from build123d import *

# Parameters (mm, degrees)
CROQUIS1_W              = 237
CROQUIS1_H              = 40
CROQUIS1_W_2            = 32.55
CROQUIS1_H_2            = 30
SALIENTE_EXTRUIR1_DEPTH = 5
SALIENTE_EXTRUIR2_DEPTH = 3
REDONDEO1_R             = 10
REDONDEO2_R             = 5


with BuildPart() as part:
    # Croquis1 → Saliente-Extruir1 (new body)
    with BuildSketch(Plane.XY):
        Polygon((254.2, -311), (254.2, -341), (284.2, -341), (284.2, -381), (314.2, -381), (314.2, -311), align=None)
        Polygon((191.65, -341), (221.65, -341), (221.65, -311), (161.65, -311), (161.65, -381), (191.65, -381), align=None)
        with Locations((243.5, -401)):
            Rectangle(CROQUIS1_W, CROQUIS1_H)
        with Locations((237.925, -326)):
            Rectangle(CROQUIS1_W_2, CROQUIS1_H_2)
    extrude(amount=SALIENTE_EXTRUIR1_DEPTH)

    # Croquis1<3> → Saliente-Extruir2 (add)
    with BuildSketch(Plane.XY):
        Polygon((254.2, -311), (254.2, -341), (284.2, -341), (284.2, -381), (314.2, -381), (314.2, -311), align=None)
        Polygon((191.65, -341), (221.65, -341), (221.65, -311), (161.65, -311), (161.65, -381), (191.65, -381), align=None)
    extrude(amount=-SALIENTE_EXTRUIR2_DEPTH)

    # Redondeo1
    redondeo1_edges = [part.edges().sort_by_distance(p)[0] for p in [
        (314.2, -381, 2.5),
        (362, -381, 2.5),
        (362, -421, 2.5),
        (125, -421, 2.5),
        (125, -381, 2.5),
        (161.65, -381, 2.5),
        (161.65, -311, 1),
        (314.2, -311, 1),
        (191.65, -381, 2.5),
        (284.2, -381, 2.5),
        (284.2, -341, 1),
        (191.65, -341, 1),
    ]]
    fillet(redondeo1_edges, radius=REDONDEO1_R)

    # Redondeo2
    redondeo2_edges = [part.edges().sort_by_distance(p)[0] for p in [
        (314.2, -381, -1.5),
        (284.2, -381, -1.5),
        (254.2, -341, -1.5),
        (254.2, -311, -1.5),
        (221.65, -341, -1.5),
        (221.65, -311, -1.5),
        (161.65, -381, -1.5),
        (191.65, -381, -1.5),
    ]]
    fillet(redondeo2_edges, radius=REDONDEO2_R)


solid = part.part
Work out the finished part from the listing and answer in its coordinate system (mm). A direction names the side the tool comes from. Round coordinates to 2 decimals unless told otherwise and drop trailing zeros. Order: outer loops, then holes, each group sorted by start corner. A loop starts at its lowest first (then second) coordinate and runs counter-clockwise, first axis right, second up. Notation, with made-up numbers: M 0.5,87.5 L 29.5,87.5 A10 ccw 29.5,101.5 Z; hole C -10,-12 d9. An arc over 180 degrees is marked long. Put each result on its own line as item: value. Start each with the question number.
Q1. Section D-D, the plane y = -408 is taken. Write down the section's boundary in (x, z), and give its area (4 significant figures).
Q2. Straight lines are drawn through the part: L1, parallel to X at y = -359, z = -2.25; L2, parallel to Y at x = 211.5, z = 1; L3, parallel to X at y = -333.5, z = -1. For each, find the intervals that lie inside material, in ascending order. Write a range as [from, to].
Q3. A tool of negligible diameter and unlimited length cuts with its end or side. For faces 1 (the cylindrical face through (190.22, -379.5, -1.52)), 2 (the cylindrical face through (358.99, -383.85, 2.54)), 3 (the cylindrical face through (281.35, -344.01, 1.06)), 4 (the flat face through (125, -401, 2)), 5 (the flat face through (143, -381, 2)), from which of +Z, -Z, +X, -X, +Y, -Y can it reach the whole face along a straight path? Write none if from no direction.
Q4. Flat-ended cylindrical pins translate along their axes: pin 1 (0.9 mm diameter, centred on y = -330.5, z = -1, fed in from -X); pin 2 (0.9 mm diameter, centred on x = 176.5, z = -1, fed in from -Y); pin 3 (1.5 mm diameter, centred on x = 343, z = 1.5, fed in from +Y). Find the tip coordinate at first contact, or state that the pin passes through.
Q5. Section B-B, the plane y = -360.5 is taken. Write down the section's boundary in (x, z).
Q6. Section C-C, the plane x = 342 is taken. Write down the section's boundary in (y, z).
Q7. For a pull along X with two mould halves and no side action, classify faces 6 (the flat face through (290, -338, -3)), 7 (the cylindrical face through (255.63, -312.5, -1.52)), 8 (the cylindrical face through (358.99, -418.15, 2.54)) as pulls with the +X half, pulls with the -X half, needs draft (parallel to the pull), parting line crosses it, or undercut.
Q8. Section A-A, the plane z = -1.5 is taken. Write down the section's boundary in (x, y), and give its area (3 significant figures).
Findings below:
1. outline: M 125,0 L 362,0 L 362,5 L 125,5 Z
1. area: 1,185 mm^2
2. L1: x = [161.65, 191.65], [284.2, 314.2]
2. L2: y = [-421, -381], [-341, -311]
2. L3: x = [161.65, 221.65], [254.2, 314.2]
3. face 1: -Z, -Y
3. face 2: +Z, -Z, +X, +Y
3. face 3: +Z, -Z
3. face 4: +Z, -Z, -X, +Y, -Y
3. face 5: +Z, -Z, -X, +Y
4. pin 1: stops at x = 161.65
4. pin 2: stops at y = -381
4. pin 3: stops at y = -381
5. outline: M 161.65,-3 L 191.65,-3 L 191.65,5 L 161.65,5 Z; M 284.2,-3 L 314.2,-3 L 314.2,5 L 284.2,5 Z
6. outline: M -421,0 L -381,0 L -381,5 L -421,5 Z
7. face 6: needs draft
7. face 7: undercut
7. face 8: pulls with the +X half
8. outline: M 161.65,-376 A5 ccw 166.65,-381 L 186.65,-381 A5 ccw 191.65,-376 L 191.65,-351 A10 cw 201.65,-341 L 216.65,-341 A5 ccw 221.65,-336 L 221.65,-316 A5 ccw 216.65,-311 L 171.65,-311 A10 ccw 161.65,-321 Z; M 254.2,-336 A5 ccw 259.2,-341 L 274.2,-341 A10 cw 284.2,-351 L 284.2,-376 A5 ccw 289.2,-381 L 309.2,-381 A5 ccw 314.2,-376 L 314.2,-321 A10 ccw 304.2,-311 L 259.2,-311 A5 ccw 254.2,-316 Z
8. area: 5,960 mm^2
